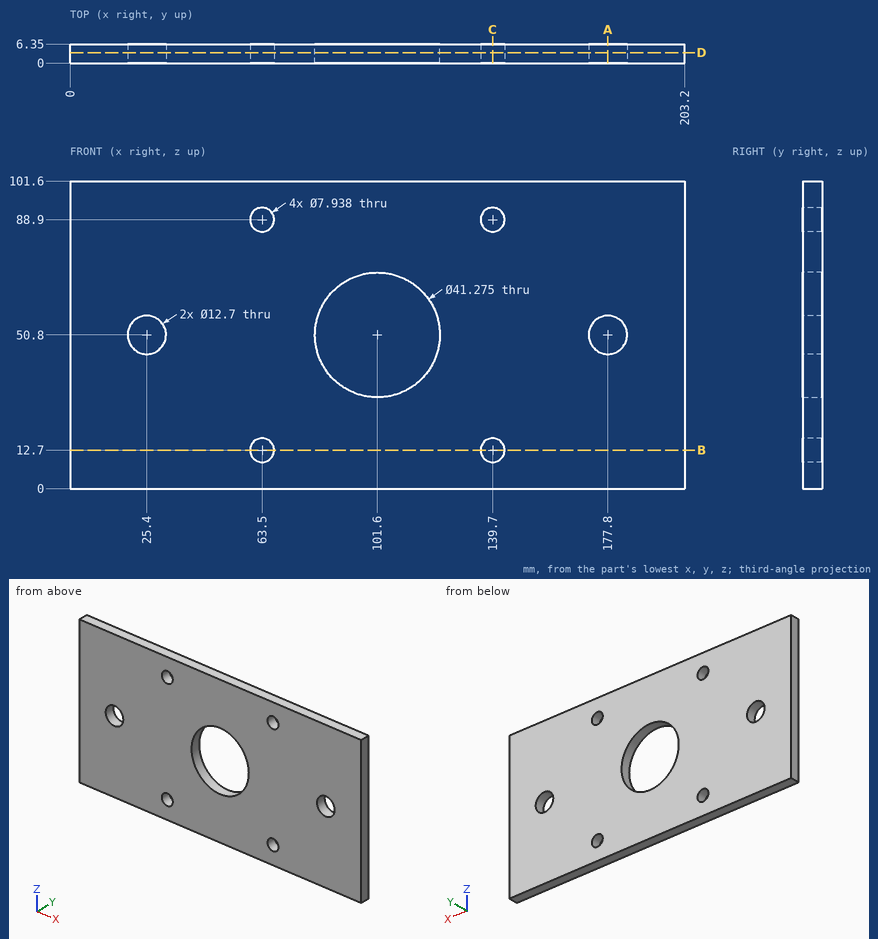
Can you work these out from the drawing? Everything is in mm from the part's minimum corner. Round coordinates to 2 decimals unless told otherwise and drop trailing zeros. Order: outer loops, then holes, each group sorted by start corner. A loop starts at its lowest first (then second) coordinate and runs counter-clockwise, first axis right, second up. Notation, with made-up numbers: (12.25, 78) - (68.25, 78) arc R15 cw to (68.25, 98) - close; hole circle Ø1 at (72.5, 3.25). An arc over 180 degrees is marked (long way). Answer in a Markdown table with one row per item.
(1) Suppose I cut it at D-D, the plane y = 3.5. Count the separate pieces of the cut face and the enclosed holes in it, plus the area to 3 significant figures.
From the geometry:
| item | result |
|---|---|
| separate pieces | 1 |
| enclosed holes | 7 |
| area | 18,900 mm2 |
(2) Suppose I cut it at C-C, the plane x = 139.7. Please give me the cut outline in (y, z).
From the geometry:
| item | result |
|---|---|
| outline | (0, 0) - (6.35, 0) - (6.35, 8.73) - (0, 8.73) - close; (0, 16.67) - (6.35, 16.67) - (6.35, 84.93) - (0, 84.93) - close; (0, 92.87) - (6.35, 92.87) - (6.35, 101.6) - (0, 101.6) - close |
(3) Suppose I cut it at A-A, the plane x = 177.8. Please give me the cut outline in (y, z).
From the geometry:
| item | result |
|---|---|
| outline | (0, 0) - (6.35, 0) - (6.35, 44.45) - (0, 44.45) - close; (0, 57.15) - (6.35, 57.15) - (6.35, 101.6) - (0, 101.6) - close |
(4) Please list where these lines run through material, in increasing order: L1, parallel to X at y = 4.25, z = 50.8; L2, parallel to X at y = 2.25, z = 88.9; L3, parallel to X at y = 3.75, z = 11 (1 decimal). Write a range as from..to.
From the geometry:
| item | result |
|---|---|
| L1 | x = 0..19.05, 31.75..80.96, 122.24..171.45, 184.15..203.2 |
| L2 | x = 0..59.53, 67.47..135.73, 143.67..203.2 |
| L3 | x = 0..59.9, 67.1..136.1, 143.3..203.2 |
(5) Suppose I cut it at B-B, the plane z = 12.7. Please give me the cut outline in (x, y), plus the area to 3 significant figures.
From the geometry:
| item | result |
|---|---|
| outline | (0, 0) - (59.53, 0) - (59.53, 6.35) - (0, 6.35) - close; (67.47, 0) - (135.73, 0) - (135.73, 6.35) - (67.47, 6.35) - close; (143.67, 0) - (203.2, 0) - (203.2, 6.35) - (143.67, 6.35) - close |
| area | 1,190 mm2 |
(6) For P1, Ø8, axis at x = 140.5, z = 25, coming from the -Y side, with a flat end and sliding along its axis, tell me the tip position at first contact or that it passes through.
From the geometry:
| item | result |
|---|---|
| P1 | stops at y = 0 |
